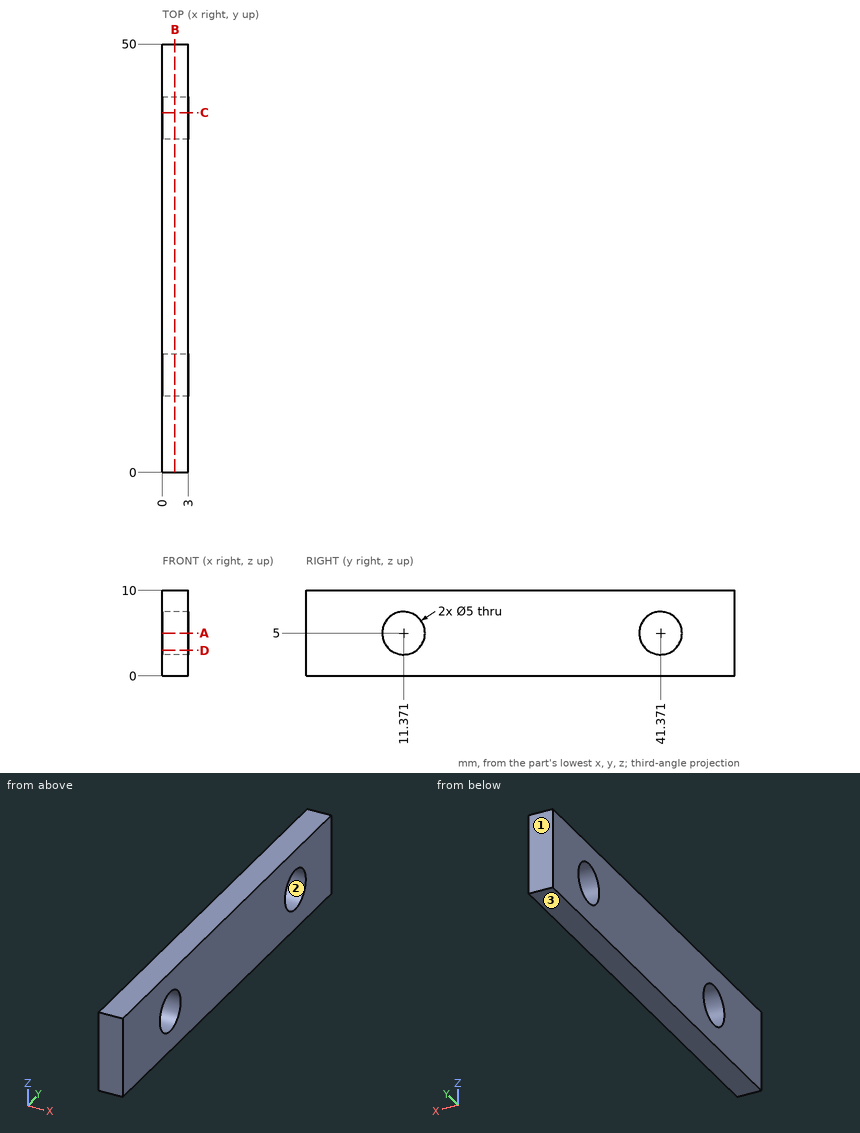
The figure shows three views and two pictorial views of one solid part (mm, origin at its lowest corner). Answer the questions. Coordinates: 2 decimals unless noted, no trailing zeros. Loops run counter-clockwise (first coordinate to the right, second up) from the corner with the lowest first, then second, coordinate; pieces in that order, holes last. Notation, with made-up numbers: M 62,45.5 L 107,45.5 A31 cw 107,71.5 Z; hole C -24,69.5 d4. An arc over 180 degrees is marked long. Answer as CSV lines item,"result". Start each with the question number.
(1) The part is cut by section A-A (z = 5). Give the vertices of the cut face in (x, y).
(2) The part is cut by section B-B (x = 1.45). Give the vertices of the cut face in (y, z), and give its area (3 significant figures).
(3) The part is cut by section C-C (y = 42). Give the vertices of the cut face in (x, z).
(4) The mould has two halves that part along Z. Classify the marked faces 1, 2 and 3: pulls with the +Z half, pulls with the -Z half, needs draft (parallel to the pull), parting line crosses it, or undercut.
(5) The part is cut by section D-D (z = 3). Give the vertices of the cut face in (x, y).
(6) Find the intervals of material crossed by L1, parallel to Y at x = 1.6, z = 6; L2, parallel to Y at x = 2.3, z = 3.25 (1 decimal); L3, parallel to Z at x = 1.05, y = 41, in increasing order. Write a range as [from, to].
Determined:
1,outline,"M 0,0 L 3,0 L 3,8.87 L 0,8.87 Z; M 0,13.87 L 3,13.87 L 3,38.87 L 0,38.87 Z; M 0,43.87 L 3,43.87 L 3,50 L 0,50 Z"
2,outline,"M 0,0 L 50,0 L 50,10 L 0,10 Z; hole C 11.37,5 d5; hole C 41.37,5 d5"
2,area,"461 mm2"
3,outline,"M 0,0 L 3,0 L 3,2.58 L 0,2.58 Z; M 0,7.42 L 3,7.42 L 3,10 L 0,10 Z"
4,face 1,"needs draft"
4,face 2,"undercut"
4,face 3,"pulls with the -Z half"
5,outline,"M 0,0 L 3,0 L 3,9.87 L 0,9.87 Z; M 0,12.87 L 3,12.87 L 3,39.87 L 0,39.87 Z; M 0,42.87 L 3,42.87 L 3,50 L 0,50 Z"
6,L1,"[0, 9.08], [13.66, 39.08], [43.66, 50]"
6,L2,"[0, 9.6], [13.2, 39.6], [43.2, 50]"
6,L3,"[0, 2.53], [7.47, 10]"
